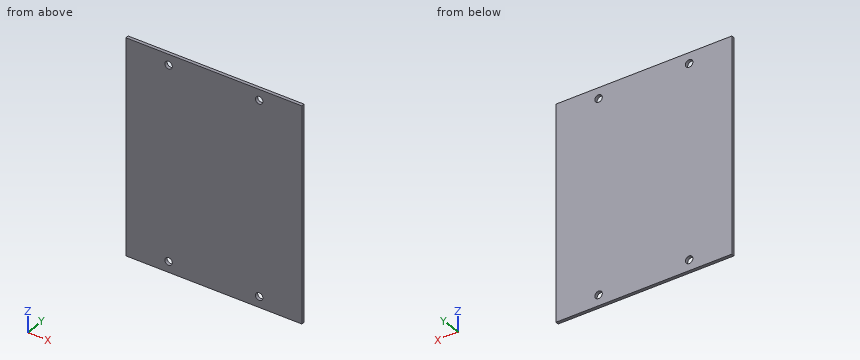
Solid Edge part; units mm, degrees
sketch "Sketch1" plane through (0, 0, 0) normal (0, -1, 0) x (1, 0, 0)
  line L0 (-82.5, -100) -> (82.5, -100)
  line L1 (82.5, -100) -> (82.5, 100)
  line L2 (82.5, 100) -> (-82.5, 100)
  line L3 (-82.5, 100) -> (-82.5, -100)
  dimension "D1" = 82.5
  dimension "D2" = 82.5
extrude "Protrusion1" add sketch "Sketch1" against normal blind 3
sketch "Sketch2" plane through (0, 0, 0) normal (0, -1, 0) x (1, 0, 0)
  circle A0 centre (-42.5, 90) radius 3.5
  circle A1 centre (42.5, 90) radius 3.5
  dimension "D1" = 42.5
extrude "Cutout1" cut sketch "Sketch2" against normal through all
sketch "Sketch3" plane through (0, 0, 0) normal (0, -1, 0) x (1, 0, 0)
  circle A0 centre (-42.5, -90) radius 3.5
  circle A1 centre (42.5, -90) radius 3.5
extrude "Cutout2" cut sketch "Sketch3" against normal through all
properties material "Nylon, allgemein"
For this review, take the finished solid that the model builds, in its own axes (mm). Give positions to 0.01 mm unless a question says otherwise; leave off trailing zeros. Loops run counter-clockwise (first coordinate to the right, second up) from the corner with the lowest first, then second, coordinate; pieces in that order, holes last. Notation, with made-up numbers: (37, 81.25) -> (95, 81.25) arc R22 cw to (95, 101.25) -> close; hole circle Ø11 at (45.5, -24). An arc over 180 degrees is marked (long way). One line per question, with ' | ' between items.
1) We need section B-B (z = 90). Write out the cut boundary in (x, y).
Resolved:
outline: (-82.5, 0) -> (-46, 0) -> (-46, 3) -> (-82.5, 3) -> close; (-39, 0) -> (39, 0) -> (39, 3) -> (-39, 3) -> close; (46, 0) -> (82.5, 0) -> (82.5, 3) -> (46, 3) -> close
2) Insertion check: pin 1 Ø9 at (x, z) = (-42.5, 90) entering from +Y. The pin has a flat end and moves straight along its axis. Give the tip position at first contact, or say it passes through.
Resolved:
pin 1: stops at y = 3
3) We need section A-A (x = 42.5). Write out the cut boundary in (y, z), plus the area to 3 significant figures.
Resolved:
outline: (0, -100) -> (3, -100) -> (3, -93.5) -> (0, -93.5) -> close; (0, -86.5) -> (3, -86.5) -> (3, 86.5) -> (0, 86.5) -> close; (0, 93.5) -> (3, 93.5) -> (3, 100) -> (0, 100) -> close | area: 558 mm2
4) To check wall thickness, follow probe 1 along Z at (x, y) = (42.5, 1.2); probe 2 along X at (y, z) = (2, -91.5). State the ranges of each line that lie inside material, in increasing order.
Resolved:
probe 1: z = -100 to -93.5, -86.5 to 86.5, 93.5 to 100 | probe 2: x = -82.5 to -45.66, -39.34 to 39.34, 45.66 to 82.5
